from build123d import *
from build123d.topology import SkipClean

# Parameters (mm, degrees)
EXTRUDE_1_DEPTH     = 35
EXTRUDE_START       = 25
EXTRUDE_3_DEPTH     = 45
EXTRUDE_4_DEPTH     = 50
SKETCH_4_W          = 20
SKETCH_4_H          = 60
CUT_EXTRUDE_1_DEPTH = 50
SKETCH_10_W         = 18
SKETCH_10_H         = 45
CUT_EXTRUDE_3_DEPTH = 60
SKETCH_12_W         = 10
SKETCH_12_H         = 12
CUT_EXTRUDE_5_DEPTH = 60


with BuildPart() as part:
    # Sketch 1 → Extrude 1 (new body)
    with BuildSketch(Plane.XY):
        Polygon((0, 0), (50, 0), (50, 20), (34, 20), (34, 11), (16, 11), (16, 19.999701213), (0, 19.999701213), align=None)
    extrude(amount=-EXTRUDE_1_DEPTH)



with BuildPart() as body_2:
    # Sketch 2 → Extrude 3 (new, symmetric)
    with SkipClean():  # the faces are left unmerged after this step: merging them gives an invalid solid
        with BuildSketch(Plane(origin=(0, 0, 0), x_dir=(0, 0, -1), z_dir=(1, 0, 0)).offset(EXTRUDE_START)):
            with BuildLine():
                ThreePointArc((20, 31.151519965), (27.5, 30), (35, 31.151519965))
                Line((35, 31.151519965), (35, 55))
                Line((35, 55), (20, 55))
                Line((20, 55), (20, 31.151519965))
            make_face()
            with BuildLine():
                Line((35, 55), (35, 31.151519965))
                ThreePointArc((35, 31.151519965), (47.655644371, 40.209800542), (52.5, 55))
                ThreePointArc((52.5, 55), (12.709800542, 75.155644371), (20, 31.151519965))
                Line((20, 31.151519965), (20, 55))
                Line((20, 55), (35, 55))
            make_face()
        extrude(amount=EXTRUDE_3_DEPTH, both=True)


with BuildPart() as part_1:
    add(part.part)

    add(body_2.part)  # Extrude 4 merges body 2
    # Sketch 3 → Extrude 4 (add)
    with BuildSketch(Plane(origin=(0, 0, 0), x_dir=(0, 0, -1), z_dir=(1, 0, 0))):
        with BuildLine():
            Line((20, 20), (35, 20))
            Line((35, 20), (35, 31.151519965))
            ThreePointArc((35, 31.151519965), (27.5, 30), (20, 31.151519965))
            Line((20, 31.151519965), (20, 20))
        make_face()
        with BuildLine():
            ThreePointArc((20, 31.151519965), (27.5, 30), (35, 31.151519965))
            Line((35, 31.151519965), (35, 55))
            Line((35, 55), (20, 55))
            Line((20, 55), (20, 31.151519965))
        make_face()
        with BuildLine():
            Line((35, 55), (35, 31.151519965))
            ThreePointArc((35, 31.151519965), (47.655644371, 40.209800542), (52.5, 55))
            ThreePointArc((52.5, 55), (12.709800542, 75.155644371), (20, 31.151519965))
            Line((20, 31.151519965), (20, 55))
            Line((20, 55), (35, 55))
        make_face()
    extrude(amount=EXTRUDE_4_DEPTH)

    # Sketch 4 → Cut-Extrude 1 (cut)
    with BuildSketch(Plane(origin=(0, 0, 0), x_dir=(0, 0, -1), z_dir=(1, 0, 0))):
        with Locations((10, 50)):
            Rectangle(SKETCH_4_W, SKETCH_4_H)
    extrude(amount=CUT_EXTRUDE_1_DEPTH, mode=Mode.SUBTRACT)

    # Sketch 10 → Cut-Extrude 3 (cut)
    with BuildSketch(Plane.XY):
        with Locations((25, 33.5)):
            Rectangle(SKETCH_10_W, SKETCH_10_H)
    extrude(amount=-CUT_EXTRUDE_3_DEPTH, mode=Mode.SUBTRACT)

    # Sketch 12 → Cut-Extrude 5 (cut)
    with BuildSketch(Plane.XY):
        with Locations((-15, 74)):
            Rectangle(SKETCH_12_W, SKETCH_12_H)
        with Locations((65, 74)):
            Rectangle(SKETCH_12_W, SKETCH_12_H)
    extrude(amount=-CUT_EXTRUDE_5_DEPTH, mode=Mode.SUBTRACT)


solid = part_1.part
CAD build for the part. Positions are in the model's coordinates, mm. A direction names the side the tool comes from. Round coordinates to 2 decimals unless told otherwise and drop trailing zeros. Write each loop counter-clockwise with the first axis right and the second up, starting at its lowest first coordinate (ties: lowest second). Pieces come first, ordered by that corner, then holes. Notation, with made-up numbers: M 3.25,-17 L 29.25,-17 A29 cw 29.25,16 Z; hole C -37,80.5 d5. An arc over 180 degrees is marked long. Use a Markdown table: item, result. Add a question column.
1. Slice it at C-C on z = -16.5. Give the cut face in (x, y).
2. Drill centre lines: probe 1 along X at (y, z) = (50, -9.5); probe 2 along Y at (x, z) = (24, -32); probe 3 along X at (y, z) = (19.5, -12). Where is each one in solid material? Low to high.
3. Flat gauge pins, fed straight in: P1, Ø8, axis at x = 11, z = -14, coming from the +Y side; P2, Ø10, axis at x = -3.5, y = 36, coming from the -Z side; P3, Ø10, axis at y = 10.5, z = -11, coming from the +X side. Where does each tip first touch, or does it go through?
4. 3-axis set-ups, long thin cutter, end or side, ignore diameter. For faces 1 (the face through (42, 20, -10)), 2 (the face through (-15, 68, -27)), 3 (the face through (24.6, 56.4, -20)), 4 (the face through (60, 73, -27)): which of +Z, -Z, +X, -X, +Y, -Y reach the whole face in a straight line?
5. Pull direction Y, two halves, no side cores. Call faces 5 (the face through (8, 20, -17)), 6 (the face through (25, 10, 0)), 7 (the face through (65, 68, -27)): released by +Y, released by -Y, zero draft, split by the parting line, or undercut.
6. Slice it at D-D on z = -47.5. Give the cut face in (x, y), then the cut area to 3 significant figures.
7. Slice it at A-A on y = 26. Give the cut face in (x, z), then the cut area to 3 significant figures.
8. Slice it at B-B on x = 11. Give the cut face in (y, z).
Reply:
| question | item | result |
|---|---|---|
| 1 | outline | M -20,32.55 L 0,32.55 L 0,77.45 L -10,77.45 L -10,68 L -20,68 Z; M 0,0 L 50,0 L 50,20 L 34,20 L 34,11 L 16,11 L 16,20 L 0,20 Z; M 50,32.55 L 70,32.55 L 70,68 L 60,68 L 60,77.45 L 50,77.45 Z |
| 2 | probe 1 | x = -20 to 0, 50 to 70 |
| 2 | probe 2 | y = 0 to 11, 56 to 79.59 |
| 2 | probe 3 | x = 0 to 16, 34 to 50 |
| 3 | P1 | stops at y = 20 |
| 3 | P2 | stops at z = -48.21 |
| 3 | P3 | stops at x = 50 |
| 4 | face 1 | +Z, +X, -X, +Y |
| 4 | face 2 | +Z, -Z, -X, +Y |
| 4 | face 3 | +Z, +Y |
| 4 | face 4 | +Z, -Z, +X, +Y |
| 5 | face 5 | undercut |
| 5 | face 6 | zero draft |
| 5 | face 7 | released by +Y |
| 6 | outline | M -20,40 L 16,40 L 16,56 L 34,56 L 34,40 L 70,40 L 70,68 L 60,68 L 60,70 L -10,70 L -10,68 L -20,68 Z |
| 6 | area | 2,370 mm^2 |
| 7 | outline | M 0,-35 L 16,-35 L 16,-20 L 0,-20 Z; M 34,-35 L 50,-35 L 50,-20 L 34,-20 Z |
| 7 | area | 480 mm^2 |
| 8 | outline | M 0,-35 L 20,-35 L 20,0 L 0,0 Z; M 20,-35 L 31.15,-35 A25 ccw 78.85,-20 L 20,-20 Z |
